Source: three-view drawing plus pictorial views. Frame: mm from the lowest corner of the part. Give positions to 0.01 mm unless a question says otherwise; leave off trailing zeros. Order: outer loops, then holes, each group sorted by start corner. A loop starts at its lowest first (then second) coordinate and runs counter-clockwise, first axis right, second up. Notation, with made-up numbers: (67, -26.75) -> (90, -26.75) arc R14 cw to (90, -9.75) -> close; hole circle Ø10 at (-2.75, 44). An arc over 180 degrees is marked (long way). Answer in a Markdown table with one row per item.
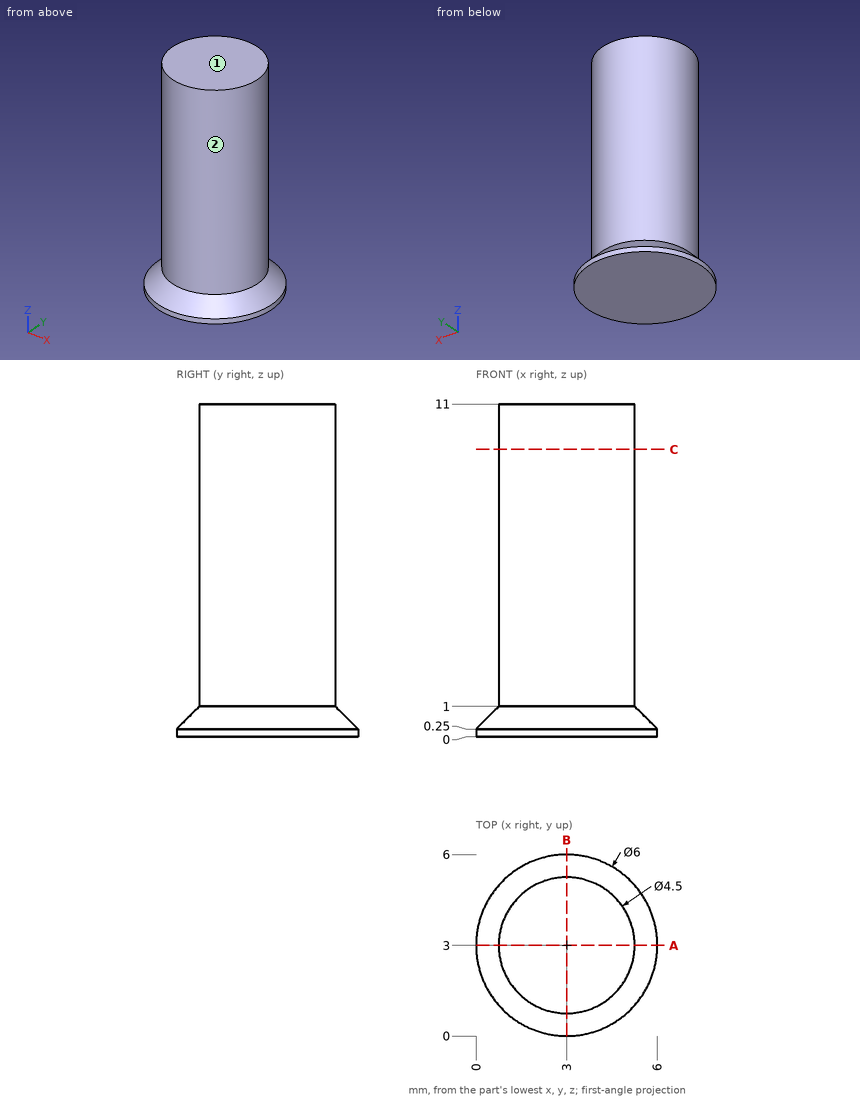
(1) Section query A-A (y = 3). Return the cut outline in (x, z), plus the area to 3 significant figures.
A:
| item | result |
|---|---|
| outline | (0, 0) -> (6, 0) -> (6, 0.25) -> (5.25, 1) -> (5.25, 11) -> (0.75, 11) -> (0.75, 1) -> (0, 0.25) -> close |
| area | 50.4 mm^2 |
(2) First-contact query: pin 1 Ø3 at (x, z) = (3, 6) entering from +Y; pin 2 Ø1.5 at (y, z) = (2.5, 1.5) entering from -X. Flat tips, straight axial feed; report the tip coordinate or a pass-through.
A:
| item | result |
|---|---|
| pin 1 | stops at y = 5.25 |
| pin 2 | stops at x = 0.54 |
(3) Section query C-C (z = 9.5). Return the cut outline in (x, y).
A:
| item | result |
|---|---|
| outline | circle Ø4.5 at (3, 3) |
(4) Ray query, probe 1 along X at (y, z) = (4.1, 7.25); probe 2 along Y at (x, z) = (2.2, 2.5); probe 3 along Y at (x, z) = (4.55, 5.25). Return the intervals inside material, ascending.
A:
| item | result |
|---|---|
| probe 1 | x = 1.04 to 4.96 |
| probe 2 | y = 0.9 to 5.1 |
| probe 3 | y = 1.37 to 4.63 |
(5) Pull-direction query (X, two-part tool) for the marked faces 1 and 2; classes: +X half, -X half, draft (parallel to the pull), parting line (faces both ways), or undercut.
A:
| item | result |
|---|---|
| face 1 | draft |
| face 2 | parting line |
